Autodesk Inventor part; units mm, degrees
ref_plane "YZ Plane" through (0, 0, 0) normal (1, 0, 0) x (0, 1, 0)
ref_plane "XZ Plane" through (0, 0, 0) normal (0, 1, 0) x (-1, 0, 0)
ref_plane "XY Plane" through (0, 0, 0) normal (0, 0, 1) x (1, 0, 0)
sketch "Sketch1" plane through (0, 0, 0) normal (0, 0, 1) x (1, 0, 0)
  line L0 (9.75, 13) -> (7.875, 9.7524)
  line L1 (7.875, 9.7524) -> (4.125, 9.7524)
  line L2 (4.125, 9.7524) -> (2.25, 13)
  line L3 (2.25, 13) -> (4.125, 16.2476)
  line L4 (4.125, 16.2476) -> (7.875, 16.2476)
  line L5 (7.875, 16.2476) -> (9.75, 13)
  point P0 (0, 0)
  point P1 (6, 13)
  dimension "d0" = 7.5
extrude "Extrusion1" add sketch "Sketch1" along normal blind 164
sketch "Sketch2" plane through (4.125, 16.2476, 0) normal (0, 1, 0) x (1, 0, 0)
  line L0 (3.75, -164) -> (5.625, -164)
  line L1 (3.75, -164) -> (0, -164)
  line L2 (0, -164) -> (-6.6597, -179.0128)
  line L3 (-1.875, 0) -> (-1.875, -164)
  line L4 (-6.6597, -191.8247) -> (-6.6597, -179.0128)
  line L5 (3.75, -164) -> (1.875, -164)
  line L6 (9.3403, -191.8668) -> (9.3403, -178.8539)
  line L7 (9.3403, -178.8539) -> (3.75, -164)
  line L8 (9.3403, -191.8668) -> (7.3403, -191.8668)
  line L9 (7.3403, -191.8668) -> (7.3403, -179.2178)
  line L10 (-6.6597, -191.8247) -> (-4.6597, -191.8247)
  line L11 (-4.6597, -191.8247) -> (-4.6597, -179.4364)
  line L12 (2.1735, -164.0436) -> (2.158, -164)
  line L13 (1.875, -175) -> (5.7529, -175)
  line L14 (-2.6917, -175) -> (1.875, -175)
  line L15 (-4.6597, -179.4364) -> (-2.6917, -175)
  line L16 (5.7529, -175) -> (7.3403, -179.2178)
  line L17 (1.875, -164) -> (1.875, -191.8247)
  point P0 (-4.125, 0)
  dimension "d12" = 2
  dimension "d13" = 2
  dimension "d16" = 27.8247
  dimension "d17" = 11
  dimension "d21" = 12
  dimension "d31" = 2
  dimension "d32" = 2
extrude "Extrusion2" add sketch "Sketch2" against normal blind 6.5
sketch "Sketch3" plane through (-2.5347, 9.7476, 179.0128) normal (-0.9141, 0, -0.4055) x (-0.4055, 0, 0.9141)
  point P0 (-164.6629, -9.7476)
sketch "Sketch5" plane through (4.125, 16.2476, 0) normal (0, 1, 0) x (1, 0, 0)
  line L0 (-1.875, -164) -> (0, -164)
  line L1 (-1.875, -164) -> (-1.875, -168.2268)
  line L2 (0, -164) -> (-6.6597, -179.0128)
  line L3 (3.75, -164) -> (5.625, -164)
  line L4 (5.625, -164) -> (5.625, -168.982)
  line L5 (9.3403, -178.8539) -> (3.75, -164)
  point P0 (-4.125, 0)
extrude "Extrusion3" add sketch "Sketch5" against normal blind 6.5
sketch "Sketch6" plane through (13.4653, 16.2476, 191.8668) normal (1, 0, 0) x (0, 0, -1)
  line L0 (0, 0) -> (0, -3.25)
  line L1 (0, 0) -> (0, -6.5)
  line L2 (0, -3.25) -> (6, -3.25)
  circle A0 centre (6, -3.25) radius 1.5
  point P0 (191.8668, -16.2476)
  dimension "d27" = 6
  dimension "d28" = 3
extrude "Extrusion4" cut sketch "Sketch6" against normal through all
sketch "Sketch7" plane through (4.125, 9.7524, 0) normal (0, -1, 0) x (1, 0, 0)
  line L0 (0, 0) -> (-6.6005, -15.1699)
  line L1 (-6.6005, -27.9818) -> (-6.6005, -15.1699)
  line L2 (9.3995, -28.0239) -> (9.3995, -15.011)
  line L3 (9.3995, -15.011) -> (3.75, 0)
  line L4 (9.3995, -28.0239) -> (7.3995, -28.0239)
  line L5 (7.3995, -28.0239) -> (7.3995, -15.3749)
  line L6 (-6.6005, -27.9818) -> (-4.6005, -27.9818)
  line L7 (-4.6005, -27.9818) -> (-4.6005, -15.5861)
  line L8 (1.9054, -10.9999) -> (5.7124, -10.8924)
  line L9 (-2.6612, -11.129) -> (1.9054, -10.9999)
  line L10 (-4.6005, -15.5861) -> (-2.6612, -11.129)
  line L11 (5.7124, -10.8924) -> (7.3995, -15.3749)
  line L12 (1.942, 0) -> (1.942, -27.8247)
  line L13 (5.625, 0) -> (3.75, 0)
  line L14 (0, 0) -> (3.75, 0)
  line L15 (3.75, 0) -> (0, 0)
  line L16 (3.75, 0) -> (0, 0)
  point P0 (-4.125, 0)
  dimension "d34" = 2
  dimension "d35" = 2
  dimension "d36" = 11
  dimension "d37" = 12
  dimension "d38" = 2
  dimension "d39" = 2
extrude "Extrusion5" add sketch "Sketch7" against normal blind 6.5
sketch "Sketch8" plane through (1.4333, 16.2476, 175) normal (0, 1, 0) x (1, 0, 0)
  line L0 (8.3167, 175) -> (6.4417, 175)
  line L1 (8.3167, 175) -> (8.3167, 179.982)
  line L2 (12.0911, 190.011) -> (6.4417, 175)
  line L3 (2.6917, 175) -> (0.8167, 175)
  line L4 (0.8167, 175) -> (0.8167, 179.3093)
  line L5 (-3.9089, 190.1699) -> (2.6917, 175)
  point P0 (-1.4333, 175)
extrude "Extrusion6" add sketch "Sketch8" against normal blind 6.5
sketch "Sketch9" plane through (13.5245, 9.7524, -15.011) normal (1, 0, 0) x (0, 0, -1)
  point P0 (-15.011, -9.7524)
sketch "Sketch10" plane through (13.5245, 9.7524, -15.011) normal (1, 0, 0) x (0, 0, -1)
  line L0 (12.9708, 0) -> (12.9708, 6.5)
  line L1 (12.9708, 3.25) -> (6.9708, 3.25)
  circle A0 centre (6.9708, 3.25) radius 1.5
  point P0 (-15.011, -9.7524)
  dimension "d44" = 6
  dimension "d45" = 3
extrude "Extrusion7" cut sketch "Sketch10" against normal through all
properties part number "Rod v1 220mm"
Check sheet for the modelled part. Datum: model origin and axes. Units: mm. A direction names the side the tool comes from. Coordinates: 2 decimals unless noted, no trailing zeros. Order: outer loops, then holes, each group sorted by start corner. A loop starts at its lowest first (then second) coordinate and runs counter-clockwise, first axis right, second up. Notation, with made-up numbers: M 45.25,-18 L 60.25,-18 A15 cw 60.25,5 Z; hole C 32.25,23 d11. An arc over 180 degrees is marked long. One line per question, with ' | ' between items. Start each with the question number.
Item 1: Sectioned sample at A-A on z = 18. Record the cut outline in (x, y) (3 decimals), and give its area (3 significant figures).
Item 2: Access from +Z, -Z, +X, -X, +Y, -Y to the whole of each face (thin tool, end or side, straight path). Record for faces 1 (the flat face through (11.634, 13.043, 173.987)), 2 (the flat face through (10.66, 13.04, 177.08)), 3 (the flat face through (5.4, 16.252, -10.7)), 4 (the flat face through (-0.476, 12, -20)), 5 (the flat face through (2.25, 13, 166)).
Item 3: Mould release check, pull along X, two halves, no side actions. Record for faces 6 (the flat face through (0.436, 13.043, 177.249)), 7 (the flat face through (5.4, 9.748, 174.6)), 8 (the flat face through (9.75, 13, -2)), 9 (the flat face through (11.524, 13, -20)): pulls with the +X half, pulls with the -X half, needs draft (parallel to the pull), parting line crosses it, or undercut.
Item 4: Gauge pin test, flat ends, axial feed: P1, Ø1.9, axis at y = 11.5, z = 187.5, coming from the +X side; P2, Ø6, axis at x = 8, z = 158, coming from the -Y side; P3, Ø2.5, axis at x = 5.5, y = 11, coming from the -Z side. Record the tip position at first contact, or that the pin passes through.
Item 5: Material ranges on line 1 (Z direction, x = -1.25, y = 13.5); line 2 (Z direction, x = 2.5, y = 10.5); line 3 (Y direction, x = 6, z = 3), recorded low to high.
Answer below:
1) outline: M 2.25,13 L 4.125,9.752 L 7.875,9.752 L 9.75,13 L 7.875,16.248 L 4.125,16.248 Z | area: 36.5 mm^2
2) face 1: +X, +Y, -Y | face 2: +Z, +Y, -Y | face 3: +Z, -Z, +X, -X, +Y | face 4: -Z, +Y, -Y | face 5: -X, +Y, -Y
3) face 6: undercut | face 7: needs draft | face 8: pulls with the +X half | face 9: undercut
4) P1: stops at x = 13.47 | P2: stops at y = 9.75 | P3: stops at z = -11.05
5) line 1: z = -27.98 to -23.4, -20.57 to -12.35, 176.12 to 184.45, 187.28 to 191.82 | line 2: z = -11.1 to 0, 164 to 175 | line 3: y = 9.75 to 16.25
